Autodesk Inventor part; units mm, degrees
ref_plane "YZ Plane" through (0, 0, 0) normal (1, 0, 0) x (0, 1, 0)
ref_plane "XZ Plane" through (0, 0, 0) normal (0, 1, 0) x (-1, 0, 0)
ref_plane "XY Plane" through (0, 0, 0) normal (0, 0, 1) x (1, 0, 0)
sketch "Sketch1" plane through (0, 0, 0) normal (0, 0, 1) x (1, 0, 0)
  line L0 (12.5, -107.2169) -> (-12.5, -107.2169)
  line L1 (-12.5, -107.2169) -> (-12.5, 107.2169)
  line L2 (-12.5, 107.2169) -> (12.5, 107.2169)
  line L3 (12.5, 107.2169) -> (12.5, -107.2169)
  line L4 (12.5, -107.2169) -> (-12.5, 107.2169) construction
  line L5 (-12.5, -107.2169) -> (12.5, 107.2169) construction
  line L6 (0, 100) -> (0, -100) construction
  line L7 (-12.5, 107.2169) -> (0, 114.4338)
  line L8 (0, 114.4338) -> (12.5, 107.2169)
  line L9 (12.5, 107.2169) -> (12.5, 92.7831)
  line L10 (12.5, 92.7831) -> (0, 85.5662)
  line L11 (0, 85.5662) -> (-12.5, 92.7831)
  line L12 (-12.5, 92.7831) -> (-12.5, 107.2169)
  line L13 (-12.5, -107.2169) -> (-12.5, -92.7831)
  line L14 (-12.5, -92.7831) -> (0, -85.5662)
  line L15 (0, -85.5662) -> (12.5, -92.7831)
  line L16 (12.5, -92.7831) -> (12.5, -107.2169)
  line L17 (12.5, -107.2169) -> (0, -114.4338)
  line L18 (0, -114.4338) -> (-12.5, -107.2169)
  line L19 (-4.2161, 101.5732) -> (4.2161, 98.4268) construction
  line L20 (-5.1425, 99.0904) -> (3.2896, 95.9441)
  line L21 (5.1425, 100.9096) -> (-3.2896, 104.0559)
  arc A0 (-3.2896, 104.0559) -> (-5.1425, 99.0904) centre (-4.2161, 101.5732) ccw
  arc A1 (3.2896, 95.9441) -> (5.1425, 100.9096) centre (4.2161, 98.4268) ccw
  circle A2 centre (0, -100) radius 4.5
  line L22 (18.5, -67.375) -> (-18.5, -67.375)
  line L23 (-18.5, -67.375) -> (-18.5, 67.375)
  line L24 (-18.5, 67.375) -> (18.5, 67.375)
  line L25 (18.5, 67.375) -> (18.5, -67.375)
  line L26 (18.5, -67.375) -> (-18.5, 67.375) construction
  line L27 (-18.5, -67.375) -> (18.5, 67.375) construction
  circle A3 centre (0, 0) radius 12.7
  point P0 (268, 0)
  point P1 (-12.5, -67.375)
  point P2 (-12.5, 67.375)
  point P3 (12.5, 67.375)
  point P4 (12.5, -67.375)
  point P5 (12.5, -2.245)
  point P6 (-12.5, -2.245)
  point P7 (-12.5, 2.245)
  point P8 (12.5, 2.245)
  dimension "d0" = 25
  dimension "d1" = 268
  dimension "d2" = 200
  dimension "d3" = 5.3
  dimension "d4" = 9
  dimension "d5" = 9
  dimension "d12" = 134.75
  dimension "d13" = 37
  dimension "d43" = 25.4
extrude "Extrusion1" add sketch "Sketch1" along normal blind 6.35 contours L17 L18 L0 | L0 L1 L14 L15 L3 | L15 L14 L1 L22 L3 | L22 L1 A3 L3 | L3 A3 L24 L25 L22 | L22 L23 L24 L1 A3 | L3 A3 | A3 L1 | A3 L1 L24 L3 | L24 L1 L11 L10 L3 | L10 L11 L1 L2 L3 | L2 L7 L8
sketch "Sketch2" plane through (0, 0, 6.35) normal (0, 0, 1) x (1, 0, 0)
  line L0 (-18.5, 67.375) -> (-18.5, -67.375)
  line L1 (-18.5, -67.375) -> (-12.5, -67.375)
  line L2 (-12.5, -67.375) -> (-12.5, -107.2169)
  line L3 (-12.5, -107.2169) -> (0, -114.4338)
  line L4 (0, -114.4338) -> (12.5, -107.2169)
  line L5 (12.5, -107.2169) -> (12.5, -67.375)
  line L6 (12.5, -67.375) -> (18.5, -67.375)
  line L7 (18.5, -67.375) -> (18.5, 67.375)
  line L8 (18.5, 67.375) -> (12.5, 67.375)
  line L9 (12.5, 67.375) -> (12.5, 107.2169)
  line L10 (12.5, 107.2169) -> (0, 114.4338)
  line L11 (0, 114.4338) -> (-12.5, 107.2169)
  line L12 (-12.5, 107.2169) -> (-12.5, 67.375)
  line L13 (-12.5, 67.375) -> (-18.5, 67.375)
  arc A0 (-3.2896, 104.0559) -> (-5.1425, 99.0904) centre (-4.2161, 101.5732) ccw
  line L14 (-3.2896, 104.0559) -> (5.1425, 100.9096)
  arc A1 (3.2896, 95.9441) -> (5.1425, 100.9096) centre (4.2161, 98.4268) ccw
  line L15 (3.2896, 95.9441) -> (-5.1425, 99.0904)
  circle A2 centre (0, -100) radius 4.5
  circle A3 centre (-13.25, 68.125) radius 1.375
  point P0 (0, 0)
  point P1 (-12.5, 69.2774)
  point P2 (-14.4024, 67.375)
  dimension "d16" = 0.75
  dimension "d17" = 2.75
  dimension "d18" = 0.75
extrude "Extrusion2" cut sketch "Sketch2" against normal through all contours L13 L12 A3 picked at (-12.4132, 68.57)
mirror "Mirror1" about plane through (0, 0, 0) normal (1, 0, 0) of "Extrusion2"
mirror "Mirror2" about plane through (0, 0, 0) normal (0, 1, 0) of "Extrusion2", "Mirror1"
sketch "Sketch3" plane through (0, 0, 6.35) normal (0, 0, 1) x (1, 0, 0)
  circle A0 centre (0, -100) radius 4.5
  arc A1 (-3.2896, 104.0559) -> (-5.1425, 99.0904) centre (-4.2161, 101.5732) ccw
  line L0 (-3.2896, 104.0559) -> (5.1425, 100.9096)
  arc A2 (3.2896, 95.9441) -> (5.1425, 100.9096) centre (4.2161, 98.4268) ccw
  line L1 (3.2896, 95.9441) -> (-5.1425, 99.0904)
  arc A3 (14.4024, -67.375) -> (12.5, -69.2774) centre (13.25, -68.125) ccw
  line L2 (14.4024, -67.375) -> (18.5, -67.375)
  line L3 (18.5, -67.375) -> (18.5, 67.375)
  line L4 (18.5, 67.375) -> (14.4024, 67.375)
  arc A4 (12.5, 69.2774) -> (14.4024, 67.375) centre (13.25, 68.125) ccw
  line L5 (12.5, 69.2774) -> (12.5, 107.2169)
  line L6 (12.5, 107.2169) -> (0, 114.4338)
  line L7 (0, 114.4338) -> (-12.5, 107.2169)
  line L8 (-12.5, 107.2169) -> (-12.5, 69.2774)
  arc A5 (-14.4024, 67.375) -> (-12.5, 69.2774) centre (-13.25, 68.125) ccw
  line L9 (-14.4024, 67.375) -> (-18.5, 67.375)
  line L10 (-18.5, 67.375) -> (-18.5, -67.375)
  line L11 (-18.5, -67.375) -> (-14.4024, -67.375)
  arc A6 (-12.5, -69.2774) -> (-14.4024, -67.375) centre (-13.25, -68.125) ccw
  line L12 (-12.5, -69.2774) -> (-12.5, -107.2169)
  line L13 (-12.5, -107.2169) -> (0, -114.4338)
  line L14 (0, -114.4338) -> (12.5, -107.2169)
  line L15 (12.5, -107.2169) -> (12.5, -69.2774)
  circle A7 centre (0, 0) radius 16 construction
  line L16 (0, 0) -> (11.3137, 11.3137) construction
  line L17 (0, 0) -> (0, 16) construction
  line L18 (0, 0) -> (0, -16) construction
  line L19 (-11.3137, -11.3137) -> (11.3137, -11.3137) construction
  line L20 (11.3137, -11.3137) -> (11.3137, 11.3137) construction
  line L21 (11.3137, 11.3137) -> (-11.3137, 11.3137) construction
  line L22 (-11.3137, 11.3137) -> (-11.3137, -11.3137) construction
  line L23 (-11.3137, -11.3137) -> (11.3137, 11.3137) construction
  line L24 (11.3137, -11.3137) -> (-11.3137, 11.3137) construction
  dimension "d21" = 32
  dimension "d22" = 45
hole "Hole1" at (-11.3137, 11.3137, 6.35) at (0, 16, 6.35) at (11.3137, 11.3137, 6.35) at (11.3137, -11.3137, 6.35) at (0, -16, 6.35) at (-11.3137, -11.3137, 6.35) direction (0, 0, -1) diameter 3.242 end through all
sketch "Sketch4" plane through (0, 0, 6.35) normal (0, 0, 1) x (1, 0, 0)
  line L0 (10, -59.375) -> (-10, -59.375) construction
  line L1 (-10, -59.375) -> (-10, 59.375) construction
  line L2 (-10, 59.375) -> (10, 59.375) construction
  line L3 (10, 59.375) -> (10, -59.375) construction
  line L4 (10, -59.375) -> (-10, 59.375) construction
  line L5 (-10, -59.375) -> (10, 59.375) construction
  line L6 (-18.5, -67.375) -> (-14.4024, -67.375) construction
  line L7 (10, -28) -> (-10, -28) construction
  line L8 (-10, -28) -> (-10, 28) construction
  line L9 (-10, 28) -> (10, 28) construction
  line L10 (10, 28) -> (10, -28) construction
  line L11 (10, -28) -> (-10, 28) construction
  line L12 (-10, -28) -> (10, 28) construction
  point P0 (0, 0)
  dimension "d30" = 20
  dimension "d32" = 8
  dimension "d44" = 56
hole "Hole2" at (-10, 59.375, 6.35) at (10, 59.375, 6.35) at (-10, -59.375, 6.35) at (10, -59.375, 6.35) at (-10, 28, 6.35) at (10, 28, 6.35) at (10, -28, 6.35) at (-10, -28, 6.35) direction (0, 0, -1) diameter 5.3 end through all
fillet "Fillet3" radius 1 18 edges at (-18.5, 67.375, 3.175) (-18.5, -67.375, 3.175) (14.4024, -67.375, 3.175) (-14.4024, -67.375, 3.175) (-12.5, -69.2774, 3.175) (18.5, -67.375, 3.175) (12.5, -69.2774, 3.175) (0, -114.4338, 3.175) (12.5, -107.2169, 3.175) (-12.5, -107.2169, 3.175) (18.5, 67.375, 3.175) (-14.4024, 67.375, 3.175) (14.4024, 67.375, 3.175) (0, 114.4338, 3.175) (-12.5, 107.2169, 3.175) (-12.5, 69.2774, 3.175) (12.5, 69.2774, 3.175) (12.5, 107.2169, 3.175)
equation "\"d18\" = d16"
properties part number "Z-Axis Nut and Bed Plate RevII" material "Aluminum 6061"
The listing builds one solid part. Answer for the finished solid, in the listing's coordinates (mm). A direction names the side the tool comes from. Coordinates: 2 decimals unless noted, no trailing zeros. Loops run counter-clockwise (first coordinate to the right, second up) from the corner with the lowest first, then second, coordinate; pieces in that order, holes last. Notation, with made-up numbers: (14.5, 80.5) -> (49.5, 80.5) arc R32 ccw to (49.5, 110.5) -> close; hole circle Ø1 at (22, 80). An arc over 180 degrees is marked (long way). Return JSON: item names as keys, results as strings. Group by question number.
(1) A cutting plane is placed at A-A on y = 28. Write down the section's boundary in (x, z), and give its area (3 significant figures).
(2) Determine the mould class of faces 1 (the flat face through (-13, 2, 6.35)), 2 (the flat face through (6.33, -110.78, 3.13)), 3 (the cylindrical face through (-6.72, 102.44, 3.13)) for opening direction Y: released by +Y, released by -Y, zero draft, split by the parting line, or undercut.
(3) A cutting plane is placed at C-C on z = 1.75. Count the separate pieces of the cut face and the enclosed holes in it, and give its area (3 significant figures).
(4) Given pin 1 Ø3 at (y, z) = (74, 3) entering from -X; pin 2 Ø2 at (x, z) = (16.5, 3) entering from +Y (3 decimals); pin 3 Ø2 at (x, z) = (-16.5, 4.5) entering from -Y (3 decimals), each flat-ended and moving along its own axis, determine where each tip first touches the part or whether it passes through.
(5) A cutting plane is placed at B-B on y = 85. Write down the section's boundary in (x, z).
(6) Find the intervals of material crossed by probe 1 along X at (y, z) = (-28, 4.75); probe 2 along Y at (x, z) = (6, 1.5); probe 3 along X at (y, z) = (3.5, 3), in increasing order. Write a range as from..to.
(7) Which of the six approach directions +Z, -Z, +X, -X, +Y, -Y give full straight-line access (tool end or side, diameter ignored) to faces 4 (the flat face through (-12.5, 88, 3)), 5 (the flat face through (12.5, -88, 3)), 6 (the cylindrical face through (-0.2, 12.7, 3.1)), 7 (the flat face through (12.5, 88, 3))?
The answers:
{
 "1": {"outline": "(-18.5, 0) -> (-12.65, 0) -> (-12.65, 6.35) -> (-18.5, 6.35) -> close; (-7.35, 0) -> (7.35, 0) -> (7.35, 6.35) -> (-7.35, 6.35) -> close; (12.65, 0) -> (18.5, 0) -> (18.5, 6.35) -> (12.65, 6.35) -> close", "area": "168 mm^2"},
 "2": {"face 1": "zero draft", "face 2": "released by -Y", "face 3": "undercut"},
 "3": {"separate pieces": "1", "enclosed holes": "17", "area": "6,280 mm^2"},
 "4": {"pin 1": "stops at x = -12.5", "pin 2": "stops at y = 67.375", "pin 3": "stops at y = -67.375"},
 "5": {"outline": "(-12.5, 0) -> (12.5, 0) -> (12.5, 6.35) -> (-12.5, 6.35) -> close"},
 "6": {"probe 1": "x = -18.5..-12.65, -7.35..7.35, 12.65..18.5", "probe 2": "y = -110.97..-11.19, 11.19..96.47, 100.39..110.97", "probe 3": "x = -18.5..-12.21, 12.21..18.5"},
 "7": {"face 4": "+Z, -Z, -X, +Y", "face 5": "+Z, -Z, +X, -Y", "face 6": "+Z, -Z", "face 7": "+Z, -Z, +X, +Y"}
}
